Design review of the part built by this model. Coordinates are the model's own, in mm. A direction names the side the tool comes from. Round coordinates to 2 decimals unless told otherwise and drop trailing zeros. Write each loop counter-clockwise with the first axis right and the second up, starting at its lowest first coordinate (ties: lowest second). Pieces come first, ordered by that corner, then holes. Notation, with made-up numbers: (68.25, 54) -> (80.25, 54) arc R19 cw to (80.25, 75) -> close; hole circle Ø10 at (-34.75, 19). An arc over 180 degrees is marked (long way). Write item = value, one per line. Start each with the question number.
Item 1: Add section A-A, the plane y = 9. State the section outline as (x, z) points, then the cut area to 3 significant figures.
Item 2: Add section C-C, the plane y = 15. State the section outline as (x, z) points, then the cut area to 3 significant figures.
Item 3: Machinability: for faces 4 (the flat face through (14, 28, -14)), 5 (the flat face through (16, 24, -20)), 6 (the flat face through (8, 16, -18)), 7 (the flat face through (35, 18, -5)), 8 (the flat face through (8, 19, -11)), which of the approach directions +Z, -Z, +X, -X, +Y, -Y give a long, thin tool a straight path to every point of the face, cutting with its end or side? Answer none if there is none.
Item 4: Add section D-D, the plane y = 5. State the section outline as (x, z) points.
Item 5: To check wall thickness, follow L1, parallel to Y at x = 33.25, z = 0; L2, parallel to Z at x = 20, y = 30.6; L3, parallel to Z at x = 0.5, y = 18. State the ranges of each line that lie inside material, in increasing order.
Item 6: Mouldability with a two-part tool opening along Y and no side actions: class faces 1 (the flat face through (32, 18, -14)), 2 (the flat face through (16, 33, 0)), 3 (the flat face through (16, 18, 20)) as released by +Y, released by -Y, zero draft, split by the parting line, or undercut.
Item 7: Add section B-B, the plane x = 16. State the section outline as (y, z) points.
Item 8: For pin 1 Ø1.2 at (y, z) = (13, -14) entering from -X; pin 2 Ø4.5 at (x, z) = (17, -13.5) entering from -Y, all flat-tipped, find the tip position at first contact; note any pin that passes through.
Autodesk Inventor part; units mm, degrees
ref_plane "YZ Plane" through (0, 0, 0) normal (1, 0, 0) x (0, 1, 0)
ref_plane "XZ Plane" through (0, 0, 0) normal (0, 1, 0) x (-1, 0, 0)
ref_plane "XY Plane" through (0, 0, 0) normal (0, 0, 1) x (1, 0, 0)
ref_plane "Work Plane13" through (0, 3, 0) normal (0, 1, 0) x (1, 0, 0)
sketch "Sketch45" plane through (0, 3, 0) normal (0, 1, 0) x (1, 0, 0)
  line L0 (35, -20) -> (-3, -20)
  line L1 (-3, -20) -> (-3, 20)
  line L2 (-3, 20) -> (35, 20)
  line L3 (35, 20) -> (35, -20)
  point P0 (0, 0)
  dimension "d142" = 38
  dimension "d143" = 40
extrude "Extrusion34" add sketch "Sketch45" along normal blind 30
sketch "Sketch46" plane through (0, 33, 0) normal (0, 1, 0) x (1, 0, 0)
  point P0 (0, 0)
ref_plane "Work Plane11" through (0, 0, 0) normal (0, -1, 0) x (1, 0, 0)
sketch "Sketch47" plane through (0, 0, 0) normal (0, -1, 0) x (1, 0, 0)
  circle A0 centre (16, 0) radius 18
  point P0 (0, 0)
  dimension "d146" = 36
extrude "Extrusion35" cut sketch "Sketch47" against normal blind 30 draft -15
sketch "Sketch48" plane through (0, 33, 0) normal (0, 1, 0) x (1, 0, 0)
  point P0 (0, 0)
sketch "Sketch49" plane through (0, 33, 0) normal (0, 1, 0) x (1, 0, 0)
  circle A0 centre (20, 0) radius 1.25
  point P0 (0, 0)
  dimension "d149" = 2.5
extrude "Extrusion36" cut sketch "Sketch49" against normal through all
ref_plane "Work Plane7" through (35, 3, -20) normal (0, 0, -1) x (-1, 0, 0)
sketch "Sketch58" plane through (35, 3, -20) normal (0, 0, -1) x (-1, 0, 0)
  line L0 (7, 20) -> (27, 20)
  line L1 (27, 20) -> (27, 5)
  line L2 (27, 5) -> (7, 5)
  line L3 (7, 5) -> (7, 20)
  point P0 (35, -3)
  dimension "d156" = 20
  dimension "d157" = 15
extrude "Extrusion38" cut sketch "Sketch58" against normal blind 15
ref_plane "Work Plane4" through (-3, 3, -20) normal (-1, 0, 0) x (0, 0, 1)
sketch "Sketch59" plane through (-3, 3, -20) normal (-1, 0, 0) x (0, 0, 1)
  line L0 (4, 25) -> (8, 25)
  line L1 (8, 25) -> (8, 5)
  line L2 (8, 5) -> (4, 5)
  line L3 (4, 5) -> (4, 25)
  point P0 (20, -3)
  dimension "d160" = 4
  dimension "d161" = 20
extrude "Extrusion39" cut sketch "Sketch59" against normal blind 35
ref_plane "Work Plane1" through (0, 3, 0) normal (0, 1, 0) x (1, 0, 0)
ref_plane "Work Plane6" through (0, 23, 0) normal (0, 1, 0) x (1, 0, 0)
sketch "Sketch62" plane through (-3, 3, -20) normal (-1, 0, 0) x (0, 0, 1)
  circle A0 centre (20, 15) radius 4
  point P0 (20, -3)
  dimension "d172" = 8
extrude "Extrusion42" cut sketch "Sketch62" against normal through all
properties part number "liquid port_only_v02"
Result set:
q1.outline = (-3, -20) -> (8, -20) -> (8, -16) -> (-3, -16) -> close; (-3, -12) -> (6.05, -12) arc R15.59 cw (long way) to (28, -9.95) -> (28, -12) -> (32, -12) -> (32, -16) -> (28, -16) -> (28, -20) -> (35, -20) -> (35, 20) -> (-3, 20) -> close
q1.area = 583 mm²
q2.outline = (-3, -20) -> (8, -20) -> (8, -16) -> (-3, -16) -> close; (-3, -12) -> (8, -12) -> (8, -11.47) arc R13.98 cw to (2.27, -2.65) -> (-3, -2.65) -> close; (-3, 2.65) -> (2.27, 2.65) arc R13.98 cw to (29.73, 2.65) -> (35, 2.65) -> (35, 20) -> (-3, 20) -> close; (28, -20) -> (35, -20) -> (35, -2.65) -> (29.73, -2.65) arc R13.98 cw to (28, -7.17) -> (28, -12) -> (32, -12) -> (32, -16) -> (28, -16) -> close
q2.area = 641 mm²
q3.face_4 = -X
q3.face_5 = -Z, +X, -X, +Y, -Y
q3.face_6 = -Z
q3.face_7 = +Z, -Z, +X, +Y, -Y
q3.face_8 = -Z, -Y
q4.outline = (-3, -20) -> (35, -20) -> (35, 20) -> (-3, 20) -> close; hole circle Ø33.32 at (16, 0)
q5.L1 = 3 to 14, 22 to 33
q5.L2 = -20 to -1.25, 1.25 to 20
q5.L3 = -20 to -16, -12 to -4, 4 to 20
q6.face_1 = undercut
q6.face_2 = released by +Y
q6.face_3 = zero draft
q7.outline = (3, -20) -> (8, -20) -> (8, -15.86) -> (3, -17.2) -> close; (3, 17.2) -> (30, 9.96) -> (30, -9.96) -> (23, -11.84) -> (23, -12) -> (28, -12) -> (28, -16) -> (23, -16) -> (23, -20) -> (33, -20) -> (33, 20) -> (3, 20) -> close
q8.pin_1 = 32
q8.pin_2 = 23
